Read the model definition and answer for the solid it produces. Units are mm, in the model's axes. Face numbers are marked on the shaded views. Give positions to 0.01 mm unless a question says otherwise; leave off trailing zeros. Order: outer loops, then holes, each group sorted by start corner. A loop starts at its lowest first (then second) coordinate and runs counter-clockwise, first axis right, second up. Notation, with made-up numbers: (-29, -13.5) - (0, -13.5) arc R22 ccw to (0, 6.5) - close; hole circle Ø3 at (29, 52.25). An arc over 180 degrees is marked (long way). Use a Markdown table: item, result. Add a question column.
1. A cutting plane is placed at C-C on z = 30. Determine the outline of the cut face in (x, y).
2. For a pull along X with two mould halves and no side action, classify the marked faces 1, 2, 3 and 4 as released by +X, released by -X, zero draft, split by the parting line, or undercut.
3. A cutting plane is placed at D-D on z = 14.5. Determine the outline of the cut face in (x, y).
4. A cutting plane is placed at B-B on x = 13. Determine the outline of the cut face in (y, z), and give its area (3 significant figures).
5. A cutting plane is placed at A-A on y = 20. Determine the outline of the cut face in (x, z).
6. Consider L1, parallel to X at y = 34, z = 30; L2, parallel to Y at x = 20.5, z = 20; L3, parallel to Z at x = 20, y = 32. Determine where each line is inside the solid, lowest interval first.
7. Flat-ended cylindrical pins translate along their axes: P1, Ø3, axis at x = 21, z = 29, coming from the +Y side; P2, Ø16, axis at x = 20, y = 20, coming from the +Z side. Find the tip coordinate at first contact, or state that the pin passes through.
```python
from build123d import *

# Parameters (mm, degrees)
ESQUISSE1_W             = 40
ESQUISSE1_H             = 40
BOSS_EXTRU_1_DEPTH      = 40
ESQUISSE2_R             = 10
ENL_V_MAT_EXTRU_1_DEPTH = 40
ESQUISSE3_R             = 5
ENL_V_MAT_EXTRU_2_DEPTH = 30


with BuildPart() as part:
    # Esquisse1 → Boss.-Extru.1 (new body)
    with BuildSketch(Plane.XY):
        with Locations((20, 20)):
            Rectangle(ESQUISSE1_W, ESQUISSE1_H)
    extrude(amount=BOSS_EXTRU_1_DEPTH)

    # Esquisse2 → Enlèv. mat.-Extru.1 (cut)
    with BuildSketch(Plane.XY.offset(40)):
        with Locations((20, 20)):
            Circle(ESQUISSE2_R)
    extrude(amount=-ENL_V_MAT_EXTRU_1_DEPTH, mode=Mode.SUBTRACT)

    # Esquisse3 → Enlèv. mat.-Extru.2 (cut)
    with BuildSketch(Plane(origin=(0, 40, 0), x_dir=(1, 0, 0), z_dir=(0, 1, 0))):
        with Locations(Location((20, -30, 0), (0, 0, 270))):
            Circle(ESQUISSE3_R)
    extrude(amount=-ENL_V_MAT_EXTRU_2_DEPTH, mode=Mode.SUBTRACT)


solid = part.part
```
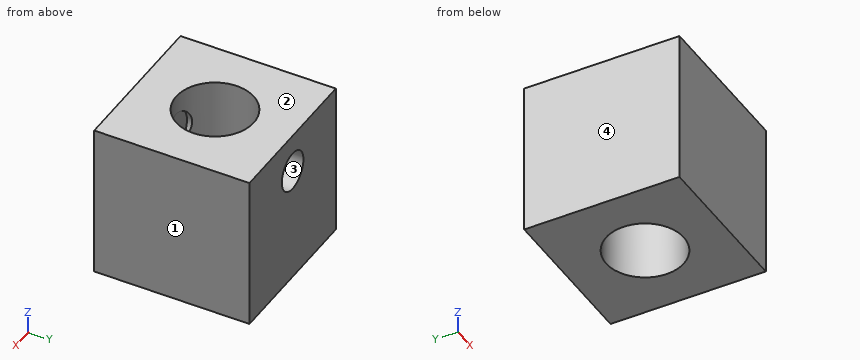
Output values:
| question | item | result |
|---|---|---|
| 1 | outline | (0, 0) - (40, 0) - (40, 40) - (25, 40) - (25, 28.66) arc R10 cw to (25, 11.34) - (25, 10) - (15, 10) - (15, 11.34) arc R10 cw to (15, 28.66) - (15, 40) - (0, 40) - close |
| 2 | face 1 | released by +X |
| 2 | face 2 | zero draft |
| 2 | face 3 | undercut |
| 2 | face 4 | released by -X |
| 3 | outline | (0, 0) - (40, 0) - (40, 40) - (0, 40) - close; hole circle Ø20 at (20, 20) |
| 4 | outline | (0, 0) - (12.86, 0) - (12.86, 40) - (0, 40) - close; (27.14, 0) - (40, 0) - (40, 40) - (27.14, 40) - close |
| 4 | area | 1,030 mm² |
| 5 | outline | (0, 0) - (10, 0) - (10, 40) - (0, 40) - close; (30, 0) - (40, 0) - (40, 40) - (30, 40) - close |
| 6 | L1 | 0 to 15, 25 to 40 |
| 6 | L2 | 0 to 10.01, 29.99 to 40 |
| 6 | L3 | 0 to 25, 35 to 40 |
| 7 | P1 | y = 10 |
| 7 | P2 | through |
